Geometry: final body of the model. Coordinates: model frame, mm. A direction names the side the tool comes from. Round coordinates to 2 decimals unless told otherwise and drop trailing zeros. Order: outer loops, then holes, each group sorted by start corner. A loop starts at its lowest first (then second) coordinate and runs counter-clockwise, first axis right, second up. Notation, with made-up numbers: M 18,-15 L 43,-15 A22 ccw 43,24 Z; hole C 38,-24 d11. An arc over 180 degrees is marked long. Put each result on its own line as item: value. Start each with the question number.
1) Material intervals for probe 1 along Y at (x, z) = (90, -83); probe 2 along Z at (x, y) = (110.5, 19); probe 3 along Y at (x, z) = (30.5, -26), sorted ascending. Write a range as [from, to].
2) Access query for faces 1 (the flat face through (79, 33, -80)), 2 (the flat face through (72, 27, 0)). Directions: +Z, -Z, +X, -X, +Y, -Y. A direction counts if a zero-diameter tool reaches every point of the face in a straight line with its end or side. Return the directions, or none.
3) Draft query along X for faces 3 (the flat face through (74, 27, -90)), 4 (the flat face through (120, 6, -44)), 5 (the cylindrical face through (93, 44, -5)). Return one class per face: pulls with the +X half, pulls with the -X half, needs draft (parallel to the pull), parting line crosses it, or undercut.
4) Section B-B, the plane y = 14. Return loops of the section in (x, z), then the cut area to 3 significant figures.
5) First-contact query: P1, Ø11.5, axis at x = 90, y = 40, coming from the +Z side; P2, Ø4, axis at x = 39.5, z = -65, coming from the +Y side. Flat tips, straight axial feed; report the tip coordinate or a pass-through.
6) Section A-A, the plane x = 108. Return loops of the section in (y, z).
7) Section C-C, the plane x = 90. Return loops of the section in (y, z), then the cut area to 3 significant figures.
8) Section D-D, the plane y = 63.5. Return loops of the section in (x, z), then the cut area to 3 significant figures.
Autodesk Inventor part; units mm, degrees
ref_plane "YZ Plane" through (0, 0, 0) normal (1, 0, 0) x (0, 1, 0)
ref_plane "XZ Plane" through (0, 0, 0) normal (0, 1, 0) x (-1, 0, 0)
ref_plane "XY Plane" through (0, 0, 0) normal (0, 0, 1) x (1, 0, 0)
sketch "Sketch1" plane through (0, 0, 0) normal (0, 1, 0) x (-1, 0, 0)
  line L0 (0, 0) -> (-120, 0)
  line L1 (-120, 0) -> (-120, -90)
  line L2 (-120, -90) -> (0, -90)
  line L3 (0, -90) -> (0, 0)
  dimension "d0" = 120
  dimension "d1" = 90
extrude "Extrusion1" add sketch "Sketch1" along normal blind 10
sketch "Sketch2" plane through (0, 10, 0) normal (0, 1, 0) x (1, 0, 0)
  point P0 (0, 0)
sketch "Sketch3" plane through (0, 10, 0) normal (0, 1, 0) x (1, 0, 0)
  line L0 (120, 0) -> (120, 90)
  line L1 (120, 0) -> (120, 10)
  line L2 (120, 10) -> (60, 10)
  line L3 (0, 0) -> (120, 0)
  line L4 (60, 10) -> (60, 0)
  line L5 (60, 0) -> (120, 0)
  line L6 (60, 0) -> (60, 90) construction
  line L7 (60, 90) -> (60, 80)
  line L8 (60, 80) -> (120, 80)
  line L9 (60, 90) -> (120, 90)
  line L10 (120, 90) -> (120, 80)
  dimension "d4" = 10
  dimension "d5" = 60
  dimension "d6" = 10
extrude "Extrusion2" add sketch "Sketch3" along normal blind 60
sketch "Sketch4" plane through (0, 0, 0) normal (0, 0, 1) x (1, 0, 0)
  line L0 (60, 10) -> (60, 70)
  line L1 (120, 0) -> (120, 70)
  line L2 (60, 70) -> (120, 70)
  line L3 (120, 70) -> (120, 20)
  line L4 (120, 20) -> (60, 20)
  line L5 (60, 20) -> (60, 70)
  circle A0 centre (90, 40) radius 30
  circle A1 centre (90, 40) radius 5
  line L6 (67.8284, 60.2094) -> (135.2299, 60.2094) construction
  line L7 (67.8284, 60.2094) -> (17.619, 10)
  line L8 (60, 10) -> (0, 10)
  line L9 (67.8284, 60.2094) -> (138.8353, 60.2094) construction
  line L10 (120, 10) -> (60, 10)
  line L11 (17.619, 10) -> (60, 10)
  line L12 (60, 10) -> (60, 40)
  point P0 (0, 0)
  point P1 (90, 70)
  point P2 (120, 40)
  dimension "d9" = 50
  dimension "d10" = 10
  dimension "d14" = 135
extrude "Extrusion3" cut sketch "Sketch4" against normal blind 100 contours L0 L7 A0 | L0 L2 A0 L7 | A0 L2 L1 | A1
extrude "Extrusion4" add sketch "Sketch4" against normal blind 90 contours L8 L7 L0 | L0 L7 A0
sketch "Sketch5" plane through (0, 0, 0) normal (1, 0, 0) x (0, 1, 0)
  line L0 (10, -10) -> (40, -10)
  line L1 (10, -10) -> (10, -80)
  line L2 (10, -10) -> (10, -80)
  line L3 (10, -80) -> (63.3463, -80)
  line L4 (63.3463, -80) -> (63.3463, -10)
  line L5 (63.3463, -10) -> (10, -10)
  point P0 (0, 0)
  dimension "d19" = 70
extrude "Extrusion5" cut sketch "Sketch5" along normal blind 90
properties part number "Foot" material "Aluminum 6061"
Result sheet:
1. probe 1: y = [0, 35], [45, 70]
1. probe 2: z = [-90, -80], [-10, 0]
1. probe 3: y = [0, 10]
2. face 1: +X, -X, +Y
2. face 2: +Z, +X, -X, +Y, -Y
3. face 3: needs draft
3. face 4: pulls with the +X half
3. face 5: undercut
4. outline: M 21.62,-90 L 120,-90 L 120,-80 L 21.62,-80 Z; M 21.62,-10 L 120,-10 L 120,0 L 21.62,0 Z
4. area: 1,970 mm2
5. P1: stops at z = 0
5. P2: stops at y = 10
6. outline: M 0,-90 L 64,-90 L 64,-80 L 10,-80 L 10,-10 L 64,-10 L 64,0 L 0,0 Z
7. outline: M 0,-90 L 35,-90 L 35,-80 L 10,-80 L 10,-10 L 35,-10 L 35,0 L 0,0 Z; M 45,-90 L 70,-90 L 70,-80 L 45,-80 Z; M 45,-10 L 70,-10 L 70,0 L 45,0 Z
7. area: 1,900 mm2
8. outline: M 71.35,-90 L 108.65,-90 L 108.65,-80 L 71.35,-80 Z; M 71.35,-10 L 108.65,-10 L 108.65,0 L 71.35,0 Z
8. area: 746 mm2
